```python
from build123d import *

# Parameters (mm, degrees)
F0_W     = 130.282268
F0_H     = 81.471775
F1_DEPTH = 100
F2_W     = 35.016233
F2_H     = 62.241167
F3_DEPTH = 100
F2_W_2   = 30.737754
F2_H_2   = 44.113887
F4_DEPTH = 100


with BuildPart() as f1:
    # F0 (on Right) → F1 (new body)
    with BuildSketch(Plane.YZ):
        with Locations((-1.179434, -2.358871)):
            Rectangle(F0_W, F0_H)
    extrude(amount=F1_DEPTH)

    # F2 (on face) → F3 (cut)
    with BuildSketch(Plane.XY.offset(38.377017)):
        with Locations((26.910903, -16.402766)):
            Rectangle(F2_W, F2_H)
    extrude(amount=-F3_DEPTH, mode=Mode.SUBTRACT)

    # F2 (on face) → F4 (cut)
    with BuildSketch(Plane.XY.offset(38.377017)):
        with Locations((74.166195, 18.735057)):
            Rectangle(F2_W_2, F2_H_2)
    extrude(amount=-F4_DEPTH, mode=Mode.SUBTRACT)


solid = f1.part
```
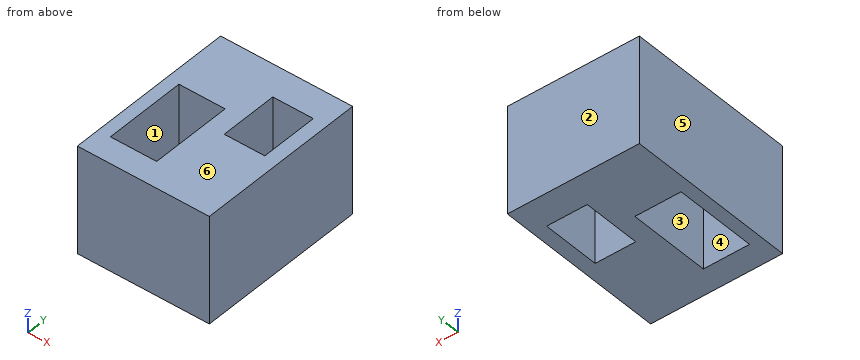
Can you work these out from the model? Positions are in its coordinate system, mm. Face numbers are marked on the shaded views. A direction names the side the tool comes from. Give positions to 0.01 mm unless a question says otherwise; leave off trailing zeros. Loops run counter-clockwise (first coordinate to the right, second up) from the corner with the lowest first, then second, coordinate; pieces in that order, holes last. Notation, with made-up numbers: M 26,68.5 L 55,68.5 A17 cw 55,93.5 Z; hole C 22,19 d7. An arc over 180 degrees is marked long. Use CSV: the item, a comma, the result in double quotes. Start each with the question number.
1. If we mould it in two halves opening along X, with no side actions, what happens to the marked faces 3, 4, 5 and 6? For each: released by +X, released by -X, zero draft, split by the parting line, or undercut.
2. Imagine slicing it at A-A, the plane y = 11.5. Write out the boundary of the cut face in (x, z).
3. Imagine slicing it at B-B, the plane z = -8. Write out the boundary of the cut face in (x, y), plus the area to 3 significant figures.
4. Imagine slicing it at C-C, the plane x = 81. Write out the boundary of the cut face in (y, z).
5. On a 3-axis mill with a long thin cutter (end or side, diameter ignored), from which of +Z, -Z, +X, -X, +Y, -Y can I reach the whole of each face in a straight line? I mean the marked faces 1 and 2. Say none if no direction works.
6. If I drill on L1, parallel to X at y = 7.5, z = 9.5; L2, parallel to Y at x = 27, z = -31.5; L3, parallel to X at y = -16.5, z = 7, over which ranges is the centre line in solid material (lowest first)?
7. Imagine slicing it at D-D, the plane y = 35. Write out the boundary of the cut face in (x, z), plus the area to 3 significant figures.
Response values:
1,face 3,"undercut"
1,face 4,"undercut"
1,face 5,"released by -X"
1,face 6,"zero draft"
2,outline,"M 0,-43.09 L 9.4,-43.09 L 9.4,38.38 L 0,38.38 Z; M 44.42,-43.09 L 58.8,-43.09 L 58.8,38.38 L 44.42,38.38 Z; M 89.54,-43.09 L 100,-43.09 L 100,38.38 L 89.54,38.38 Z"
3,outline,"M 0,-66.32 L 100,-66.32 L 100,63.96 L 0,63.96 Z; hole M 9.4,-47.52 L 44.42,-47.52 L 44.42,14.72 L 9.4,14.72 Z; hole M 58.8,-3.32 L 89.54,-3.32 L 89.54,40.79 L 58.8,40.79 Z"
3,area,"9,490 mm^2"
4,outline,"M -66.32,-43.09 L -3.32,-43.09 L -3.32,38.38 L -66.32,38.38 Z; M 40.79,-43.09 L 63.96,-43.09 L 63.96,38.38 L 40.79,38.38 Z"
5,face 1,"+Z, -Z"
5,face 2,"+Z, -Z, +X, -X, +Y"
6,L1,"0 to 9.4, 44.42 to 58.8, 89.54 to 100"
6,L2,"-66.32 to -47.52, 14.72 to 63.96"
6,L3,"0 to 9.4, 44.42 to 100"
7,outline,"M 0,-43.09 L 58.8,-43.09 L 58.8,38.38 L 0,38.38 Z; M 89.54,-43.09 L 100,-43.09 L 100,38.38 L 89.54,38.38 Z"
7,area,"5,640 mm^2"
